from build123d import *

# Parameters (mm, degrees)
SKETCH1_W           = 42
SKETCH1_H           = 20.5
BOSS_EXTRUDE1_DEPTH = 39.5
SKETCH2_W           = 5.185118418
SKETCH2_H           = 20.5
SKETCH2_R           = 1.27
SKETCH2_W_2         = 5.144602193
BOSS_EXTRUDE2_DEPTH = 5.08


with BuildPart() as part:
    # Sketch1 → Boss-Extrude1 (new body)
    with BuildSketch(Plane.XY):
        with Locations((21, 10.25)):
            Rectangle(SKETCH1_W, SKETCH1_H)
    extrude(amount=BOSS_EXTRUDE1_DEPTH)

    # Sketch2 → Boss-Extrude2 (add)
    with BuildSketch(Plane(origin=(0, 0, 28.448), x_dir=(-1, 0, 0), z_dir=(0, 0, -1))):
        with Locations((2.592559209, 10.25)):
            Rectangle(SKETCH2_W, SKETCH2_H)
        with Locations((3.5, 5.25)):
            Circle(SKETCH2_R, mode=Mode.SUBTRACT)
        with Locations((3.5, 15.25)):
            Circle(SKETCH2_R, mode=Mode.SUBTRACT)
        with Locations((-44.572301096, 10.25)):
            Rectangle(SKETCH2_W_2, SKETCH2_H)
        with Locations((-45.5, 5.25)):
            Circle(SKETCH2_R, mode=Mode.SUBTRACT)
        with Locations((-45.5, 15.25)):
            Circle(SKETCH2_R, mode=Mode.SUBTRACT)
    extrude(amount=-BOSS_EXTRUDE2_DEPTH)


solid = part.part
Design review of the part built by this model. Coordinates are the model's own, in mm. A direction names the side the tool comes from. Round coordinates to 2 decimals unless told otherwise and drop trailing zeros. Write each loop counter-clockwise with the first axis right and the second up, starting at its lowest first coordinate (ties: lowest second). Pieces come first, ordered by that corner, then holes. Notation, with made-up numbers: (-38, 18.25) - (1, 18.25) arc R13 cw to (1, 28.25) - close; hole circle Ø10 at (59.25, -27.5). An arc over 180 degrees is marked (long way). Use a Markdown table: item, result. Add a question column.
1. Wall thickness on probe 1 along Y at (x, z) = (-3.5, 30.8); probe 2 along X at (y, z) = (11, 25.5); probe 3 along Y at (x, z) = (-3, 31): over which ranges is each line inside the solid? List them lowest first.
2. We need section B-B (y = 15.25). State the section outline as (x, z) points.
3. Mouldability with a two-part tool opening along Y and no side actions: class faces 5 (the face through (21, 20.5, 19)), 6 (the face through (42, 10, 36)), 7 (the face through (21, 0, 19)), 8 (the face through (45.78, 4.01, 30.95)) as +Y half, -Y half, draft (parallel to the pull), parting line (faces both ways), or undercut.
4. For faces 1 (the face through (0, 10, 14)), 2 (the face through (42, 10, 14)), 3 (the face through (45, 10, 33.528)), 4 (the face through (0, 10, 36)), list the 3-axis set-ups (+Z, -Z, +X, -X, +Y, -Y) from which the entire face can be reached by the end or side of a thin tool; tool diameter is ignored.
5. We need section C-C (z = 30). State the section outline as (x, y) points.
6. We need section D-D (y = 12.25). State the section outline as (x, z) points.
7. Clearance check with flat-ended pins moving along their axes: pin 1 (4 mm diameter, centred on x = -3.5, y = 11.5, fed in from -Z); pin 2 (3.5 mm diameter, centred on x = -3.5, y = 15.25, fed in from +Z); pin 3 (12 mm diameter, centred on x = 18, y = 2, fed in from -Z); pin 4 (1.5 mm diameter, centred on x = 45.5, y = 15.25, fed in from -Z). State where each tip first meets the part, or that it passes through.
8. We need section A-A (x = -3.5). State the section outline as (y, z) points.
Output:
| question | item | result |
|---|---|---|
| 1 | probe 1 | y = 0 to 3.98, 6.52 to 13.98, 16.52 to 20.5 |
| 1 | probe 2 | x = 0 to 42 |
| 1 | probe 3 | y = 0 to 4.08, 6.42 to 14.08, 16.42 to 20.5 |
| 2 | outline | (-5.19, 28.45) - (-4.77, 28.45) - (-4.77, 33.53) - (-5.19, 33.53) - close; (-2.23, 28.45) - (0, 28.45) - (0, 0) - (42, 0) - (42, 28.45) - (44.23, 28.45) - (44.23, 33.53) - (42, 33.53) - (42, 39.5) - (0, 39.5) - (0, 33.53) - (-2.23, 33.53) - close; (46.77, 28.45) - (47.14, 28.45) - (47.14, 33.53) - (46.77, 33.53) - close |
| 3 | face 5 | +Y half |
| 3 | face 6 | draft |
| 3 | face 7 | -Y half |
| 3 | face 8 | undercut |
| 4 | face 1 | -Z, -X, +Y, -Y |
| 4 | face 2 | -Z, +X, +Y, -Y |
| 4 | face 3 | +Z, +X, +Y, -Y |
| 4 | face 4 | +Z, -X, +Y, -Y |
| 5 | outline | (-5.19, 0) - (47.14, 0) - (47.14, 20.5) - (-5.19, 20.5) - close; hole circle Ø2.54 at (-3.5, 5.25); hole circle Ø2.54 at (-3.5, 15.25); hole circle Ø2.54 at (45.5, 5.25); hole circle Ø2.54 at (45.5, 15.25) |
| 6 | outline | (-5.19, 28.45) - (0, 28.45) - (0, 0) - (42, 0) - (42, 28.45) - (47.14, 28.45) - (47.14, 33.53) - (42, 33.53) - (42, 39.5) - (0, 39.5) - (0, 33.53) - (-5.19, 33.53) - close |
| 7 | pin 1 | stops at z = 28.45 |
| 7 | pin 2 | stops at z = 33.53 |
| 7 | pin 3 | stops at z = 0 |
| 7 | pin 4 | passes through |
| 8 | outline | (0, 28.45) - (3.98, 28.45) - (3.98, 33.53) - (0, 33.53) - close; (6.52, 28.45) - (13.98, 28.45) - (13.98, 33.53) - (6.52, 33.53) - close; (16.52, 28.45) - (20.5, 28.45) - (20.5, 33.53) - (16.52, 33.53) - close |
